from build123d import *

# Parameters (mm, degrees)
SKETCH1_W           = 28.575
SKETCH1_H           = 26.9875
SKETCH1_W_2         = 22.479
SKETCH1_H_2         = 22.479
BOSS_EXTRUDE1_DEPTH = 31.75
FILLET1_R           = 5.08
SKETCH2_R           = 2.38125
BOSS_EXTRUDE2_DEPTH = 3.96875
SKETCH3_R           = 2.38125
BOSS_EXTRUDE3_DEPTH = 2.38125
FILLET2_R           = 4.7625
FILLET3_R           = 4.7625


with BuildPart() as part:
    # Sketch1 → Boss-Extrude1 (new body, symmetric)
    with BuildSketch(Plane(origin=(0, 0, 0), x_dir=(0, 0, -1), z_dir=(1, 0, 0))):
        Rectangle(SKETCH1_W, SKETCH1_H)
        Rectangle(SKETCH1_W_2, SKETCH1_H_2, mode=Mode.SUBTRACT)
    extrude(amount=BOSS_EXTRUDE1_DEPTH, both=True)

    # Fillet1
    fillet1_edges = [part.edges().sort_by_distance(p)[0] for p in [
        (0, -11.2395, -11.2395),
        (0, 11.2395, -11.2395),
        (0, 11.2395, 11.2395),
        (0, -11.2395, 11.2395),
    ]]
    fillet(fillet1_edges, radius=FILLET1_R)

    # Sketch2 → Boss-Extrude2 (add, symmetric)
    with BuildSketch(Plane.XY):
        with BuildLine():
            Line((7.553126188, 13.49375), (9.159515278, 19.488875702))
            ThreePointArc((9.159515278, 19.488875702), (11.378487026, 22.380695986), (14.992362728, 22.856471748))
            Line((14.992362728, 22.856471748), (27.043500936, 19.627378997))
            ThreePointArc((27.043500936, 19.627378997), (30.437793711, 17.359385074), (31.75, 13.49375))
            Line((31.75, 13.49375), (7.553126188, 13.49375))
        make_face()
        with Locations((13.759737026, 18.25625)):
            Circle(SKETCH2_R, mode=Mode.SUBTRACT)
    extrude(amount=BOSS_EXTRUDE2_DEPTH, both=True)

    # Sketch3 → Boss-Extrude3 (add, symmetric)
    with BuildSketch(Plane.XY):
        with BuildLine():
            ThreePointArc((-31.75, 19.05), (-30.197271921, 22.198621069), (-26.754061915, 22.883518123))
            Line((-26.754061915, 22.883518123), (7.602422382, 13.677725901))
            Line((7.602422382, 13.677725901), (7.553126188, 13.49375))
            Line((7.553126188, 13.49375), (-31.75, 13.49375))
            Line((-31.75, 13.49375), (-31.75, 19.05))
        make_face()
        with Locations((-27.78125, 19.05)):
            Circle(SKETCH3_R, mode=Mode.SUBTRACT)
    extrude(amount=BOSS_EXTRUDE3_DEPTH, both=True)

    # Fillet2
    fillet2_edges = [part.edges().sort_by_distance(p)[0] for p in [
        (7.602422382, 13.677725901, 0),
    ]]
    fillet(fillet2_edges, radius=FILLET2_R)

    # Fillet3
    fillet3_edges = [part.edges().sort_by_distance(p)[0] for p in [
        (7.553126188, 13.49375, 3.175),
        (7.553126188, 13.49375, -3.175),
    ]]
    fillet(fillet3_edges, radius=FILLET3_R)


solid = part.part
Design review of the part built by this model. Coordinates are the model's own, in mm. A direction names the side the tool comes from. Round coordinates to 2 decimals unless told otherwise and drop trailing zeros. Write each loop counter-clockwise with the first axis right and the second up, starting at its lowest first coordinate (ties: lowest second). Pieces come first, ordered by that corner, then holes. Notation, with made-up numbers: (-18, 19) -> (7, 19) arc R27 ccw to (7, 52) -> close; hole circle Ø3 at (-19.5, -33.75). An arc over 180 degrees is marked (long way). One line per question, with ' | ' between items.
(1) Wall thickness on line 1 (Y direction, x = 28, z = 6.25); line 2 (Z direction, x = 6.5, y = -1); line 3 (Y direction, x = -3.5, z = -1.75): over which ranges is each line inside the solid? List them lowest first. Write a range as [from, to].
Result sheet:
line 1: [-13.49, -11.24], [11.24, 13.49] | line 2: [-14.29, -11.24], [11.24, 14.29] | line 3: [-13.49, -11.24], [11.24, 16.65]
(2) Draft analysis for pull direction X (two halves, no side actions). For faces 4 (the flat face through (31.75, -12, 0)), 5 (the cylindrical face through (6.66, 15.41, -0.03)), 6 (the flat face through (8.898, 18.513, 0.056)), 7 (the flat face through (21, 17, 3.969)), state which applies: released by +X, released by -X, zero draft, split by the parting line, or undercut.
Result sheet:
face 4: released by +X | face 5: undercut | face 6: undercut | face 7: zero draft
(3) Take a section at C-C, the plane x = 12.5. State the section outline as (y, z) points.
Result sheet:
outline: (-13.49, -14.29) -> (13.49, -14.29) -> (13.49, -3.97) -> (16.24, -3.97) -> (16.24, 3.97) -> (13.49, 3.97) -> (13.49, 14.29) -> (-13.49, 14.29) -> close; (20.28, -3.97) -> (22.85, -3.97) -> (22.85, 3.97) -> (20.28, 3.97) -> close; hole (-11.24, -6.16) arc R5.08 ccw to (-6.16, -11.24) -> (6.16, -11.24) arc R5.08 ccw to (11.24, -6.16) -> (11.24, 6.16) arc R5.08 ccw to (6.16, 11.24) -> (-6.16, 11.24) arc R5.08 ccw to (-11.24, 6.16) -> close
(4) Take a section at D-D, the plane y = -2. State the section outline as (x, z) points, and give its area (3 significant figures).
Result sheet:
outline: (-31.75, -14.29) -> (31.75, -14.29) -> (31.75, -11.24) -> (-31.75, -11.24) -> close; (-31.75, 11.24) -> (31.75, 11.24) -> (31.75, 14.29) -> (-31.75, 14.29) -> close | area: 387 mm2
(5) Take a section at A-A, the plane z = 4.75. State the section outline as (x, y) points, and give its area (3 significant figures).
Result sheet:
outline: (-31.75, -13.49) -> (31.75, -13.49) -> (31.75, -11.24) -> (-31.75, -11.24) -> close; (-31.75, 11.24) -> (31.75, 11.24) -> (31.75, 13.49) -> (-31.75, 13.49) -> close | area: 286 mm2
(6) Take a section at B-B, the plane z = -3.25. State how many separate pieces and enclosed holes the cut face has, and give its area (3 significant figures).
Result sheet:
separate pieces: 2 | enclosed holes: 1 | area: 442 mm2
(7) Insertion check: P1, Ø3.5, axis at x = -0.5, z = -2.5, coming from the +Y side; P2, Ø3.5, axis at x = -10.5, z = 5.5, coming from the +Y side; P3, Ø5, axis at x = -3, y = 16.5, coming from the -Z side. Each pin has a flat end and moves straight along its axis. Give the tip position at first contact, or say it passes through.
Result sheet:
P1: y = 16.32 | P2: y = 13.49 | P3: z = -2.38
(8) Machinability: for faces 1 (the cylindrical face through (6.832, 14.505, -3.164)), 2 (the flat face through (0, -11.24, 0)), 3 (the flat face through (-16, 17, 2.381)), which of the approach directions +Z, -Z, +X, -X, +Y, -Y give a long, thin tool a straight path to every point of the face, cutting with its end or side? Answer none if there is none.
Result sheet:
face 1: -Z, -X, +Y | face 2: +X, -X | face 3: +Z, -X, +Y
